Check sheet for the modelled part. Datum: model origin and axes. Units: mm. Coordinates: 2 decimals unless noted, no trailing zeros. Write each loop counter-clockwise with the first axis right and the second up, starting at its lowest first coordinate (ties: lowest second). Pieces come first, ordered by that corner, then holes. Notation, with made-up numbers: M -5,35 L 21,35 A16 ccw 21,40 Z; hole C -22,2.25 d7. An arc over 180 degrees is marked long. Answer as CSV lines item,"result". Start each with the question number.
1) Draft check along X on faces 1 (the cylindrical face through (-1.163, -304.445, 22.378)), 2 (the flat face through (-38.604, -158, 17)), 3 (the flat face through (-1, -158, 30.542)), 4 (the cylindrical face through (-1.163, -4.815, 22.378)). Enter one of: +X half, -X half, draft (parallel to the pull), parting line (faces both ways), or undercut.
2) Material ranges on L1, parallel to Y at x = 29, z = 23; L2, parallel to Y at x = -9, z = 26.75; L3, parallel to Z at x = 9.5, y = -229, recorded low to high. Write a range as [from, to].
3) Go/stop test with a flat-tipped pin: pin 1 Ø6.5 at (y, z) = (-88.19, 22.49) entering from +X. Record where the tip stops, or that it passes through.
4) Section check C-C (x = 17). Record the cut outline in (y, z), and give its area (3 significant figures).
5) Section check A-A (x = 0). Record the cut outline in (y, z).
6) Section check B-B (y = -90.5). Record the cut outline in (x, z), and give its area (3 significant figures).
from build123d import *

# Parameters (mm, degrees)
F0_W     = 75.557
F0_H     = 16.102
F1_DEPTH = 313
F2_R     = 5.336
F3_DEPTH = 75.558
F4_DEPTH = 4
F5_DEPTH = 3
F6_R     = 5.363
F7_DEPTH = 25
F8_R     = 5.363
F9_DEPTH = 25


with BuildPart() as f1:
    # F0 (on Front) → F1 (new body)
    with BuildSketch(Plane.XZ):
        with Locations((-0.825944015, 22.4905000767)):
            Rectangle(F0_W, F0_H)
    extrude(amount=F1_DEPTH)

    # F2 (on face) → F3 (cut, through all)
    with BuildSketch(Plane(origin=(-38.604444015, 0, 0), x_dir=(0, -1, 0), z_dir=(-1, 0, 0))):
        with Locations((18.192, 22.4905000767)):
            Circle(F2_R)
        with Locations((88.192, 22.4905000767)):
            Circle(F2_R)
        with Locations((158.192, 22.4905000767)):
            Circle(F2_R)
        with Locations((228.192, 22.4905000767)):
            Circle(F2_R)
        with Locations((298.192, 22.4905000767)):
            Circle(F2_R)
    extrude(amount=-F3_DEPTH, mode=Mode.SUBTRACT)

    # F4 (add): a face of the model
    f4_faces = [f1.faces().sort_by_distance(p)[0] for p in [
        (-0.825944015, -313, 22.4905000767),
    ]]
    extrude(f4_faces, amount=F4_DEPTH)

    # F5 (cut): a face of the model
    f5_faces = [f1.faces().sort_by_distance(p)[0] for p in [
        (-0.825944015, 0, 22.4905000767),
    ]]
    extrude(f5_faces, amount=-F5_DEPTH, mode=Mode.SUBTRACT)

    # F6 (on face) → F7 (cut)
    with BuildSketch(Plane(origin=(0, 0, 14.4395000767), x_dir=(1, 0, 0), z_dir=(0, 0, -1))):
        with Locations((0, 309.6801936626)):
            Circle(F6_R)
    extrude(amount=-F7_DEPTH, mode=Mode.SUBTRACT)

    # F8 (on face) → F9 (cut)
    with BuildSketch(Plane(origin=(0, 0, 14.4395000767), x_dir=(1, 0, 0), z_dir=(0, 0, -1))):
        with Locations((0, 10.0503147011)):
            Circle(F8_R)
    extrude(amount=-F9_DEPTH, mode=Mode.SUBTRACT)


solid = f1.part
Results found:
1,face 1,"undercut"
1,face 2,"-X half"
1,face 3,"draft"
1,face 4,"undercut"
2,L1,"y = [-317, -303.5], [-292.88, -233.5], [-222.88, -163.5], [-152.88, -93.5], [-82.88, -23.5], [-12.88, -3]"
2,L2,"y = [-317, -301.41], [-294.98, -231.41], [-224.98, -161.41], [-154.98, -91.41], [-84.98, -21.41], [-14.98, -3]"
2,L3,"z = [14.44, 17.22], [27.76, 30.54]"
3,pin 1,"passes through"
4,outline,"M -317,14.44 L -3,14.44 L -3,30.54 L -317,30.54 Z; hole C -298.19,22.49 d10.67; hole C -228.19,22.49 d10.67; hole C -158.19,22.49 d10.67; hole C -88.19,22.49 d10.67; hole C -18.19,22.49 d10.67"
4,area,"4,610 mm2"
5,outline,"M -317,14.44 L -315.04,14.44 L -315.04,30.54 L -317,30.54 Z; M -304.32,14.44 L -15.41,14.44 L -15.41,17.94 A5.34 cw long -15.41,27.05 L -15.41,30.54 L -304.32,30.54 Z; M -4.69,14.44 L -3,14.44 L -3,30.54 L -4.69,30.54 Z; hole C -298.19,22.49 d10.67; hole C -228.19,22.49 d10.67; hole C -158.19,22.49 d10.67; hole C -88.19,22.49 d10.67"
6,outline,"M -38.6,14.44 L 36.95,14.44 L 36.95,17.68 L -38.6,17.68 Z; M -38.6,27.3 L 36.95,27.3 L 36.95,30.54 L -38.6,30.54 Z"
6,area,"490 mm2"
